Part model, mm, in its own coordinate system. Give positions to 0.01 mm unless a question says otherwise; leave off trailing zeros. Write each loop counter-clockwise with the first axis right and the second up, starting at its lowest first coordinate (ties: lowest second). Pieces come first, ordered by that corner, then holes. Notation, with made-up numbers: (-14, -28.75) - (42, -28.75) arc R29 cw to (42, -3.75) - close; hole circle Ø7 at (-12.5, -30.75). An arc over 180 degrees is marked (long way). Answer as a JSON object with one key per item and string values. Group by question number.
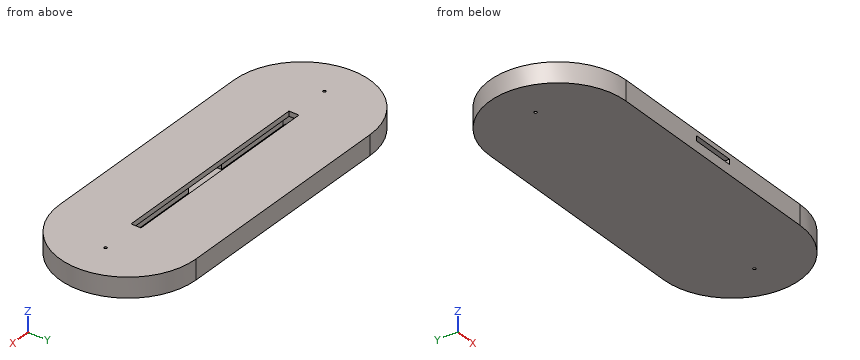
```python
from build123d import *

# Parameters (mm, degrees)
PAD_DEPTH          = 9
POCKET_DEPTH       = 6
SKETCH002_W        = 26.5
SKETCH002_H        = 35
POCKET001_DEPTH    = 6
SKETCH003_W        = 127
SKETCH003_H        = 6
PAD001_DEPTH       = 3
SKETCH004_R        = 0.85
POCKET002_DEPTH    = 485.929265
POLARPATTERN_COUNT = 2
SKETCH005_W        = 26.5
SKETCH005_H        = 7.5
PAD002_DEPTH       = 3


with BuildPart() as part:
    # Sketch → Pad (new body)
    with BuildSketch(Plane.XY):
        with BuildLine():
            ThreePointArc((-70, 41), (-111, 0), (-70, -41))
            Line((-70, -41), (70, -41))
            ThreePointArc((70, -41), (111, 0), (70, 41))
            Line((-70, 41), (70, 41))
        make_face()
    extrude(amount=PAD_DEPTH)

    # Sketch001 (on Face6 of Pad) → Pocket (cut)
    with BuildSketch(Plane.XY.offset(9)):
        with BuildLine():
            ThreePointArc((-62.5, 6), (-68.5, 0), (-62.5, -6))
            Line((-62.5, -6), (62.5, -6))
            ThreePointArc((62.5, -6), (68.5, 0), (62.5, 6))
            Line((-62.5, 6), (62.5, 6))
        make_face()
    extrude(amount=-POCKET_DEPTH, mode=Mode.SUBTRACT)

    # Sketch002 (on Face5 of Pocket) → Pocket001 (cut)
    with BuildSketch(Plane.XY.offset(9)):
        with Locations((0, -23.5)):
            Rectangle(SKETCH002_W, SKETCH002_H)
    extrude(amount=-POCKET001_DEPTH, mode=Mode.SUBTRACT)

    # Sketch003 (on Face5 of Pocket001) → Pad001 (join)
    with BuildSketch(Plane.XY.offset(9)):
        with BuildLine():
            ThreePointArc((-70, 41), (-111, 0), (-70, -41))
            Line((-70, -41), (70, -41))
            ThreePointArc((70, -41), (111, 0), (70, 41))
            Line((-70, 41), (70, 41))
        make_face()
        Rectangle(SKETCH003_W, SKETCH003_H, mode=Mode.SUBTRACT)
    extrude(amount=PAD001_DEPTH)

    # Sketch004 (on Face12 of Pad001) → Pocket002 (cut, through all)
    with BuildSketch(Plane.XY.offset(12)):
        with Locations((-88, 0)):
            Circle(SKETCH004_R)
    pocket002 = extrude(amount=-POCKET002_DEPTH, mode=Mode.SUBTRACT)

    # PolarPattern: Pocket002 ×2 about axis
    polarpattern_axis = Axis((0, 0, 12), (0, 0, 1))
    for i in range(1, POLARPATTERN_COUNT):
        add(pocket002.rotate(polarpattern_axis, i * 360 / POLARPATTERN_COUNT), mode=Mode.SUBTRACT)

    # Sketch005 (on Face10 of PolarPattern) → Pad002 (join)
    with BuildSketch(Plane.XY.offset(3)):
        with Locations((0, -37.25)):
            Rectangle(SKETCH005_W, SKETCH005_H)
    extrude(amount=PAD002_DEPTH)


solid = part.part
```
1) Saw through at D-D (y = 16.5). List the corners of the cut face in (x, z).
2) Saw through at C-C (x = 39.5). List the corners of the cut face in (y, z).
3) Saw through at B-B (y = -11.5). List the corners of the cut face in (x, z), and give its area (3 significant figures).
4) Saw through at A-A (x = -0.5). List the corners of the cut face in (y, z).
5) Drill centre lines: line 1 along Y through (x, z) = (55.5, 8.5); line 2 along Z through (x, y) = (66.5, 3.5); line 3 along Y through (x, z) = (-88, 7). Where is each one in solid material? Low to high. Write a range as from..to.
6) Drop flat-ended pins along their axis: P1, Ø2.5, axis at y = 0, z = 11, coming from the +X side; P2, Ø1.5, axis at x = 88, y = 0, coming from the -Z side; P3, Ø3, axis at y = -30, z = 5, coming from the -X side; P4, Ø3, axis at y = -13, z = 8.5, coming from the +X side. Give the stop position or say it passes through.
Checks:
{
 "1": {"outline": "(-107.53, 0) - (107.53, 0) - (107.53, 12) - (-107.53, 12) - close"},
 "2": {"outline": "(-41, 0) - (41, 0) - (41, 12) - (3, 12) - (3, 9) - (6, 9) - (6, 3) - (-6, 3) - (-6, 9) - (-3, 9) - (-3, 12) - (-41, 12) - close"},
 "3": {"outline": "(-109.35, 0) - (109.35, 0) - (109.35, 12) - (-109.35, 12) - close; hole (-13.25, 3) - (13.25, 3) - (13.25, 9) - (-13.25, 9) - close", "area": "2,470 mm2"},
 "4": {"outline": "(-41, 0) - (41, 0) - (41, 12) - (3, 12) - (3, 9) - (6, 9) - (6, 3) - (-33.5, 3) - (-33.5, 6) - (-41, 6) - close; (-41, 9) - (-3, 9) - (-3, 12) - (-41, 12) - close"},
 "5": {"line 1": "-41..-6, 6..41", "line 2": "0..3, 9..12", "line 3": "-36.84..-0.85, 0.85..36.84"},
 "6": {"P1": "x = 111", "P2": "through", "P3": "x = -99.47", "P4": "x = 109.35"}
}
